Input: part model. Units: mm. Frame: model coordinates. Coordinates: 2 decimals unless noted, no trailing zeros. Order: outer loops, then holes, each group sorted by start corner. A loop starts at its lowest first (then second) coordinate and runs counter-clockwise, first axis right, second up. Notation, with made-up numbers: (-1.75, -39) - (52.25, -39) arc R32 ccw to (52.25, -4) - close; hole circle Ø4 at (35, -9.5). An arc over 180 degrees is marked (long way). One line per question, with ' | ' between items. Start each with the question number.
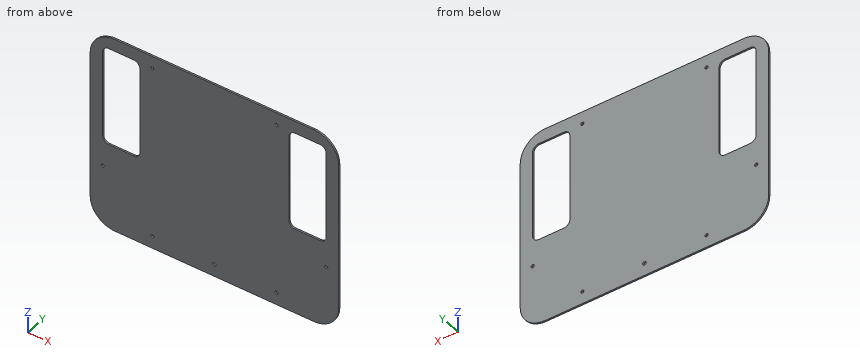
```python
from build123d import *

# Parameters (mm, degrees)
SKETCH1_W                       = 508
SKETCH1_H                       = 406.4
EXTRUDE1_DEPTH                  = 3.175
SKETCH2_W                       = 76.2
SKETCH2_H                       = 203.2
EXTRUDE2_DEPTH                  = 326.294206258
FILLET2_R                       = 50.8
FILLET3_R                       = 12.7
F_1_4_0_25_DIAMETER_HOLE1_D     = 6.35
F_1_4_0_25_DIAMETER_HOLE1_DEPTH = 25.4
F_1_4_0_25_DIAMETER_HOLE1_TIP   = 1.907732465
CUT_EXTRUDE1_REACH              = 327.294
SKETCH5_R                       = 3.57844787


with BuildPart() as part:
    # Sketch1 → Extrude1 (new body)
    with BuildSketch(Plane(origin=(0, 0, 0), x_dir=(1, 0, 0), z_dir=(0, 1, 0))):
        Rectangle(SKETCH1_W, SKETCH1_H)
    extrude(amount=EXTRUDE1_DEPTH)

    # Sketch2 → Extrude2 (cut, through all)
    with BuildSketch(Plane(origin=(0, 3.175, 0), x_dir=(1, 0, 0), z_dir=(0, 1, 0))):
        with Locations((-190.5, -76.2)):
            Rectangle(SKETCH2_W, SKETCH2_H)
        with Locations((190.5, -76.2)):
            Rectangle(SKETCH2_W, SKETCH2_H)
    extrude(amount=-EXTRUDE2_DEPTH, mode=Mode.SUBTRACT)

    # Fillet2
    fillet2_edges = [part.edges().sort_by_distance(p)[0] for p in [
        (-254, 1.5875, -203.2),
        (254, 1.5875, -203.2),
        (254, 1.5875, 203.2),
        (-254, 1.5875, 203.2),
    ]]
    fillet(fillet2_edges, radius=FILLET2_R)

    # Fillet3
    fillet3_edges = [part.edges().sort_by_distance(p)[0] for p in [
        (-228.6, 1.5875, 177.8),
        (-228.6, 1.5875, -25.4),
        (-152.4, 1.5875, -25.4),
        (-152.4, 1.5875, 177.8),
        (152.4, 1.5875, 177.8),
        (152.4, 1.5875, -25.4),
        (228.6, 1.5875, -25.4),
        (228.6, 1.5875, 177.8),
    ]]
    fillet(fillet3_edges, radius=FILLET3_R)

    # 1/4 (0.25) Diameter Hole1
    with Locations(Plane(origin=(0, 3.175, 0), x_dir=(-1, 0, 0), z_dir=(0, 1, 0))):
        with Locations((127, -177.8), (-127, -177.8), (-228.6, -76.2), (228.6, -76.2), (127, 177.8), (-127, 177.8)):
            Hole(F_1_4_0_25_DIAMETER_HOLE1_D / 2, depth=F_1_4_0_25_DIAMETER_HOLE1_DEPTH)
            with Locations((0, 0, -(F_1_4_0_25_DIAMETER_HOLE1_DEPTH + F_1_4_0_25_DIAMETER_HOLE1_TIP / 2))):  # 118° drill point
                Cone(0, F_1_4_0_25_DIAMETER_HOLE1_D / 2, F_1_4_0_25_DIAMETER_HOLE1_TIP, mode=Mode.SUBTRACT)

    # Sketch5 → Cut-Extrude1 (cut, up to next)
    with BuildSketch(Plane(origin=(0, 3.175, 0), x_dir=(1, 0, 0), z_dir=(0, 1, 0)), mode=Mode.PRIVATE) as cut_extrude1_sk1:
        with Locations(Location((0, 177.8, 0), (0, 0, 270))):
            Circle(SKETCH5_R)
    cut_extrude1_tool1 = extrude(cut_extrude1_sk1.sketch, amount=-CUT_EXTRUDE1_REACH, mode=Mode.PRIVATE) & part.part
    add(cut_extrude1_tool1.solids().sort_by_distance((0, 3.175, -177.8))[0], mode=Mode.SUBTRACT)


solid = part.part
```
(1) Material intervals for line 1 along Z through (x, y) = (-127, 2.3) (3 decimals); line 2 along X through (y, z) = (1.2, 53); line 3 along Z through (x, y) = (-200.5, 1.9), sorted ascending. Write a range as from..to.
(2) Pin query (flat end, axial travel): pin 1 (5.5 mm diameter, centred on x = 127, z = 177.8, fed in from +Y). Return the tip coordinate at first contact, or that it passes through.
(3) Section B-B (z = 6). Output: boundary loops of the cut face in (x, y) (3 decimals).
(4) Section A-A (y = 1.4). State how many separate pieces and enclosed holes the cut face has, then the cut area to 3 significant figures.
Worked answers:
1) line 1: z = -203.2..-180.975, -174.625..174.625, 180.975..203.2 | line 2: x = -254..-228.6, -152.4..152.4, 228.6..254 | line 3: z = -203.2..-25.4, 177.8..203.2
2) pin 1: passes through
3) outline: (-254, 0) - (-228.6, 0) - (-228.6, 3.175) - (-254, 3.175) - close; (-152.4, 0) - (152.4, 0) - (152.4, 3.175) - (-152.4, 3.175) - close; (228.6, 0) - (254, 0) - (254, 3.175) - (228.6, 3.175) - close
4) separate pieces: 1 | enclosed holes: 9 | area: 173,000 mm²
